Part model, mm, in its own coordinate system. Round coordinates to 2 decimals unless told otherwise and drop trailing zeros. Order: outer loops, then holes, each group sorted by start corner. A loop starts at its lowest first (then second) coordinate and runs counter-clockwise, first axis right, second up. Notation, with made-up numbers: (68.25, 12.5) -> (92.25, 12.5) arc R18 cw to (92.25, 27.5) -> close; hole circle Ø9 at (-6, -16). An arc over 180 degrees is marked (long way). Answer as a JSON object with one key per item and string values. Group by question number.
```python
from build123d import *

# Parameters (mm, degrees)
SKETCH1_W           = 100
SKETCH1_H           = 100
BOSS_EXTRUDE1_DEPTH = 2.5
SKETCH5_W           = 80
SKETCH5_H           = 80
CUT_EXTRUDE2_DEPTH  = 4
SKETCH6_R           = 15
BOSS_EXTRUDE3_DEPTH = 2.5
SKETCH7_W           = 5
SKETCH7_H           = 5
CUT_EXTRUDE3_DEPTH  = 2.5
BOSS_EXTRUDE4_DEPTH = 2.5
EXTRUDE_THIN2_DEPTH = 2.5
SKETCH10_R          = 3
CUT_EXTRUDE5_DEPTH  = 2.5
SKETCH12_R          = 10
CUT_EXTRUDE7_DEPTH  = 10


with BuildPart() as part:
    # Sketch1 → Boss-Extrude1 (new body)
    with BuildSketch(Plane(origin=(0, 0, 0), x_dir=(1, 0, 0), z_dir=(0, 1, 0))):
        Rectangle(SKETCH1_W, SKETCH1_H)
    extrude(amount=BOSS_EXTRUDE1_DEPTH)

    # Sketch5 → Cut-Extrude2 (cut)
    with BuildSketch(Plane(origin=(0, 2.5, 0), x_dir=(1, 0, 0), z_dir=(0, 1, 0))):
        Rectangle(SKETCH5_W, SKETCH5_H)
    extrude(amount=-CUT_EXTRUDE2_DEPTH, mode=Mode.SUBTRACT)

    # Sketch8 → Boss-Extrude4 (add)
    with BuildSketch(Plane(origin=(0, 2.5, 0), x_dir=(1, 0, 0), z_dir=(0, 1, 0))):
        with BuildLine():
            Line((-40, -40), (-27.220069463, -40))
            ThreePointArc((-27.220069463, -40), (-30.963224454, -30.963224454), (-40, -27.220069463))
            Line((-40, -27.220069463), (-40, -40))
        make_face()
        with BuildLine():
            ThreePointArc((-40, 27.220069463), (-30.963224454, 30.963224454), (-27.220069463, 40))
            Line((-27.220069463, 40), (-40, 40))
            Line((-40, 40), (-40, 27.220069463))
        make_face()
        with BuildLine():
            Line((40, 40), (27.220069463, 40))
            ThreePointArc((27.220069463, 40), (30.963224454, 30.963224454), (40, 27.220069463))
            Line((40, 27.220069463), (40, 40))
        make_face()
        with BuildLine():
            ThreePointArc((40, -27.220069463), (30.963224454, -30.963224454), (27.220069463, -40))
            Line((27.220069463, -40), (40, -40))
            Line((40, -40), (40, -27.220069463))
        make_face()
    extrude(amount=-BOSS_EXTRUDE4_DEPTH)



with BuildPart() as body_2:
    # Sketch6 → Boss-Extrude3 (new body)
    with BuildSketch(Plane(origin=(0, 2.5, 0), x_dir=(1, 0, 0), z_dir=(0, 1, 0))):
        with Locations(Location((0, 0, 0), (0, 0, 270))):
            Circle(SKETCH6_R)
    extrude(amount=-BOSS_EXTRUDE3_DEPTH)

    # Sketch7 → Cut-Extrude3 (cut)
    with BuildSketch(Plane(origin=(0, 2.5, 0), x_dir=(1, 0, 0), z_dir=(0, 1, 0))):
        Rectangle(SKETCH7_W, SKETCH7_H)
    extrude(amount=-CUT_EXTRUDE3_DEPTH, mode=Mode.SUBTRACT)


with BuildPart() as part_1:
    add(part.part)

    add(body_2.part)  # Extrude-Thin2 merges body 2
    # Sketch9 → Extrude-Thin2 (add)
    with BuildSketch(Plane(origin=(0, 2.5, 0), x_dir=(1, 0, 0), z_dir=(0, 1, 0))):
        Polygon((-1.035533906, -6.035533906), (34.46870341, -41.539771222), (41.539771222, -34.46870341), (6.035533906, 1.035533906), align=None)
        Polygon((-11.285533906, -4.214466094), (-41.539771222, -34.46870341), (-34.46870341, -41.539771222), (-4.214466094, -11.285533906), align=None)
        Polygon((11.285533906, 4.214466094), (41.539771222, 34.46870341), (34.46870341, 41.539771222), (4.214466094, 11.285533906), align=None)
        Polygon((-4.214466094, 11.285533906), (-34.46870341, 41.539771222), (-41.539771222, 34.46870341), (-11.285533906, 4.214466094), align=None)
    extrude(amount=-EXTRUDE_THIN2_DEPTH)

    # Sketch10 → Cut-Extrude5 (cut)
    with BuildSketch(Plane(origin=(0, 2.5, 0), x_dir=(1, 0, 0), z_dir=(0, 1, 0))):
        with Locations(Location((36, 36, 0), (0, 0, 270))):
            Circle(SKETCH10_R)
        with Locations(Location((-36, 36, 0), (0, 0, 90))):
            Circle(SKETCH10_R)
        with Locations(Location((36, -36, 0), (0, 0, 90))):
            Circle(SKETCH10_R)
        with Locations(Location((-36, -36, 0), (0, 0, 270))):
            Circle(SKETCH10_R)
    extrude(amount=-CUT_EXTRUDE5_DEPTH, mode=Mode.SUBTRACT)

    # Sketch12 → Cut-Extrude7 (cut)
    with BuildSketch(Plane(origin=(0, 2.5, 0), x_dir=(1, 0, 0), z_dir=(0, 1, 0))):
        with Locations(Location((0, 0, 0), (0, 0, 270))):
            Circle(SKETCH12_R)
    extrude(amount=-CUT_EXTRUDE7_DEPTH, mode=Mode.SUBTRACT)


solid = part_1.part
```
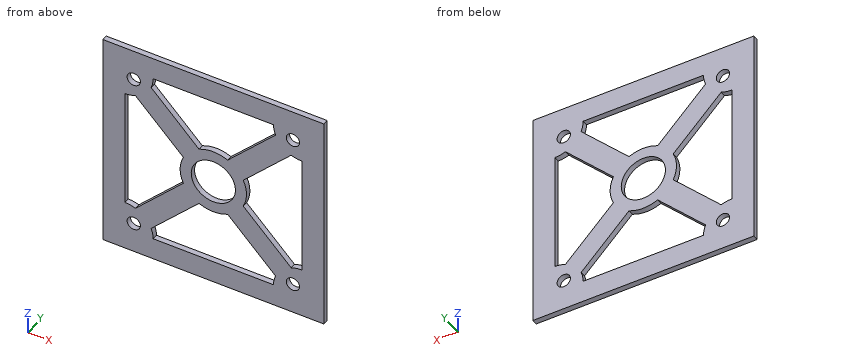
Q1. Band-saw the part on D-D (x = 0). List the corners of the cut face in (y, z), plus the area to 3 significant figures.
Q2. Band-saw the part on B-B (x = 30). List the corners of the cut face in (y, z).
Q3. Band-saw the part on C-C (z = 4). List the corners of the cut face in (x, y), plus the area to 3 significant figures.
Q4. Band-saw the part on A-A (y = 0.75). Count the separate pieces of the cut face and the enclosed holes in it, plus the area to 3 significant figures.
Q5. Drop a flat-ended pin along its axis: pin 1 Ø3.5 at (x, z) = (-36, 36) entering from -Y. Give the stop position or say it passes through.
Q6. Wall check: line 1 (Z direction, x = -0.5, y = 1.1); line 2 (X direction, y = 0.7, z = -22.5); line 3 (Z direction, x = -18.5, y = 2.3). Give the ranges that are in metal, low to high. Write a range as [from, to].
Completed:
{
 "1": {"outline": "(0, -50) -> (2.5, -50) -> (2.5, -40) -> (0, -40) -> close; (0, -15) -> (2.5, -15) -> (2.5, -10) -> (0, -10) -> close; (0, 10) -> (2.5, 10) -> (2.5, 15) -> (0, 15) -> close; (0, 40) -> (2.5, 40) -> (2.5, 50) -> (0, 50) -> close", "area": "75.0 mm2"},
 "2": {"outline": "(0, -50) -> (2.5, -50) -> (2.5, -22.93) -> (0, -22.93) -> close; (0, 22.93) -> (2.5, 22.93) -> (2.5, 50) -> (0, 50) -> close"},
 "3": {"outline": "(-50, 0) -> (-40, 0) -> (-40, 2.5) -> (-50, 2.5) -> close; (-14.46, 0) -> (-9.17, 0) -> (-9.17, 2.5) -> (-14.46, 2.5) -> close; (9.17, 0) -> (14.46, 0) -> (14.46, 2.5) -> (9.17, 2.5) -> close; (40, 0) -> (50, 0) -> (50, 2.5) -> (40, 2.5) -> close", "area": "76.5 mm2"},
 "4": {"separate pieces": "1", "enclosed holes": "9", "area": "5,570 mm2"},
 "5": {"pin 1": "through"},
 "6": {"line 1": "[-50, -40], [-14.99, -9.99], [9.99, 14.99], [40, 50]", "line 2": "[-50, -40], [-29.57, -15.43], [15.43, 29.57], [40, 50]", "line 3": "[-50, -40], [-25.57, -11.43], [11.43, 25.57], [40, 50]"}
}
